Source: CAD feature listing. Evaluate the final solid. Frame: model axes, mm. A direction names the side the tool comes from. Give positions to 0.01 mm unless a question says otherwise; leave off trailing zeros. Order: outer loops, then holes, each group sorted by start corner. A loop starts at its lowest first (then second) coordinate and runs counter-clockwise, first axis right, second up. Notation, with made-up numbers: M 24,69 L 39,69 A22 cw 39,108 Z; hole C 40,-40 d1. An arc over 180 degrees is marked long. Return JSON: item names as keys, results as strings.
from build123d import *

# Parameters (mm, degrees)
SKETCH1_W           = 431.8
SKETCH1_H           = 304.8
BOSS_EXTRUDE1_DEPTH = 12.7
SKETCH2_W           = 63.5
SKETCH2_H           = 12.7
SKETCH2_W_2         = 76.2
CUT_EXTRUDE1_DEPTH  = 265.574866531


with BuildPart() as part:
    # Sketch1 → Boss-Extrude1 (new body)
    with BuildSketch(Plane(origin=(0, 0, 0), x_dir=(0, 0, -1), z_dir=(1, 0, 0))):
        Rectangle(SKETCH1_W, SKETCH1_H)
    extrude(amount=BOSS_EXTRUDE1_DEPTH)

    # Sketch2 → Cut-Extrude1 (cut, through all)
    with BuildSketch(Plane(origin=(12.7, 0, 0), x_dir=(0, 0, -1), z_dir=(1, 0, 0))):
        with Locations((-184.15, 146.05)):
            Rectangle(SKETCH2_W, SKETCH2_H)
        with Locations((-38.1, 146.05)):
            Rectangle(SKETCH2_W_2, SKETCH2_H)
        with Locations((114.3, 146.05)):
            Rectangle(SKETCH2_W_2, SKETCH2_H)
    extrude(amount=-CUT_EXTRUDE1_DEPTH, mode=Mode.SUBTRACT)


solid = part.part
1. Ray query, probe 1 along Y at (x, z) = (11.5, 168). Return the intervals inside material, ascending.
Evaluation:
{"probe 1": "y = -152.4 to 139.7"}
2. Section query A-A (x = 5). Return loops of the section in (y, z).
Evaluation:
{"outline": "M -152.4,-215.9 L 152.4,-215.9 L 152.4,-152.4 L 139.7,-152.4 L 139.7,-76.2 L 152.4,-76.2 L 152.4,0 L 139.7,0 L 139.7,76.2 L 152.4,76.2 L 152.4,152.4 L 139.7,152.4 L 139.7,215.9 L -152.4,215.9 Z"}
3. First-contact query: pin 1 (3 mm diameter, centred on y = 6.5, z = -34, fed in from -X); pin 2 (4 mm diameter, centred on x = 4, y = 149, fed in from +Z). Flat tips, straight axial feed; report the tip coordinate or a pass-through.
Evaluation:
{"pin 1": "stops at x = 0", "pin 2": "stops at z = 152.4"}
4. Section query B-B (z = 172.5). Return loops of the section in (x, y).
Evaluation:
{"outline": "M 0,-152.4 L 12.7,-152.4 L 12.7,139.7 L 0,139.7 Z"}
5. Set-up query: faces 4 (the face through (0, 2, 3)), 5 (the face through (6, 139.7, -114)), 6 (the face through (6, 139.7, 185)). Return all of +Z, -Z, +X, -X, +Y, -Y with unobstructed straight access to the full face (end or side cutting, diameter ignored); none if empty.
Evaluation:
{"face 4": "+Z, -Z, -X, +Y, -Y", "face 5": "+X, -X, +Y", "face 6": "+Z, +X, -X, +Y"}
6. Draft query along Z for faces 1 (the face through (6, -2, -215.9)), 2 (the face through (6, 152.4, -38)), 3 (the face through (6, 146, 76.2)). Return one class per face: pulls with the +Z half, pulls with the -Z half, needs draft (parallel to the pull), parting line crosses it, or undercut.
Evaluation:
{"face 1": "pulls with the -Z half", "face 2": "needs draft", "face 3": "undercut"}
